```python
from build123d import *

# Parameters (mm, degrees)
BOSS_EXTRUDE1_DEPTH                       = 1.0668
CSK_FOR_6_FLAT_HEAD_MACHINE_SCREW_2_COUNT = 2
CSK_FOR_6_FLAT_HEAD_MACHINE_SCREW_2_PITCH = 75.64076181
CSK_FOR_6_FLAT_HEAD_MACHINE_SCREW_3_COUNT = 2
CSK_FOR_6_FLAT_HEAD_MACHINE_SCREW_3_PITCH = 28.085742046
CSK_FOR_6_FLAT_HEAD_MACHINE_SCREW_4_COUNT = 2
CSK_FOR_6_FLAT_HEAD_MACHINE_SCREW_4_PITCH = 31.783974209
CSK_FOR_6_FLAT_HEAD_MACHINE_SCREW_5_COUNT = 2
CSK_FOR_6_FLAT_HEAD_MACHINE_SCREW_5_PITCH = 85.183025791
CSK_FOR_6_FLAT_HEAD_MACHINE_SCREW_6_COUNT = 2
CSK_FOR_6_FLAT_HEAD_MACHINE_SCREW_6_PITCH = 53.560025791
CUT_EXTRUDE1_DEPTH                        = 78.375632316


with BuildPart() as part:
    # Sketch1 → Boss-Extrude1 (new body)
    with BuildSketch(Plane.XY):
        Polygon((-55.191374672, 13.731073684), (-72.605702167, -16.431426316), (75.603297833, -16.431426316), (58.188970339, 13.731073684), align=None)
    extrude(amount=BOSS_EXTRUDE1_DEPTH)

    # Sketch2 → CSK for #6 Flat Head Machine Screw (100)1 (revolve, cut)
    with BuildSketch(Plane(origin=(28.278810729, -11.668926316, 0), x_dir=(0, 1, 0), z_dir=(1, 0, 0))):
        Polygon((0, 0), (0, 1.0668), (1.89865, 1.0668), (1.89865, 1.380025208), (3.5433, 0), align=None)
    csk_for_6_flat_head_machine_screw_100 = revolve(axis=Axis((28.278810729, -11.668926316, -6.35), (0, 0, 1)), mode=Mode.SUBTRACT)

    # CSK for _6 Flat Head Machine Screw _ 2: CSK for #6 Flat Head Machine Screw (100)1 ×2
    with Locations(*[Vector(-0.9620606437367123, 0.27283569739479224, 0) * (i * CSK_FOR_6_FLAT_HEAD_MACHINE_SCREW_2_PITCH) for i in range(1, CSK_FOR_6_FLAT_HEAD_MACHINE_SCREW_2_COUNT)]):
        add(csk_for_6_flat_head_machine_screw_100, mode=Mode.SUBTRACT)

    # CSK for _6 Flat Head Machine Screw _ 3: CSK for #6 Flat Head Machine Screw (100)1 ×2
    with Locations(*[Vector(0.6782801027330659, 0.7348034446274878, 0) * (i * CSK_FOR_6_FLAT_HEAD_MACHINE_SCREW_3_PITCH) for i in range(1, CSK_FOR_6_FLAT_HEAD_MACHINE_SCREW_3_COUNT)]):
        add(csk_for_6_flat_head_machine_screw_100, mode=Mode.SUBTRACT)

    # CSK for _6 Flat Head Machine Screw _ 4: CSK for #6 Flat Head Machine Screw (100)1 ×2
    with Locations(*[(i * CSK_FOR_6_FLAT_HEAD_MACHINE_SCREW_4_PITCH, 0, 0) for i in range(1, CSK_FOR_6_FLAT_HEAD_MACHINE_SCREW_4_COUNT)]):
        add(csk_for_6_flat_head_machine_screw_100, mode=Mode.SUBTRACT)

    # CSK for _6 Flat Head Machine Screw _ 5: CSK for #6 Flat Head Machine Screw (100)1 ×2
    with Locations(*[(-i * CSK_FOR_6_FLAT_HEAD_MACHINE_SCREW_5_PITCH, 0, 0) for i in range(1, CSK_FOR_6_FLAT_HEAD_MACHINE_SCREW_5_COUNT)]):
        add(csk_for_6_flat_head_machine_screw_100, mode=Mode.SUBTRACT)

    # CSK for _6 Flat Head Machine Screw _ 6: CSK for #6 Flat Head Machine Screw (100)1 ×2
    with Locations(*[(-i * CSK_FOR_6_FLAT_HEAD_MACHINE_SCREW_6_PITCH, 0, 0) for i in range(1, CSK_FOR_6_FLAT_HEAD_MACHINE_SCREW_6_COUNT)]):
        add(csk_for_6_flat_head_machine_screw_100, mode=Mode.SUBTRACT)

    # Sketch4 → Cut-Extrude1 (cut, through all)
    with BuildSketch(Plane(origin=(0, 0, 0), x_dir=(-1, 0, 0), z_dir=(0, 0, -1))):
        Polygon((-65.308634086, 1.399454341), (-63.933818758, 0.605704341), (-56.355883234, 13.731073684), (-58.188970339, 13.731073684), align=None)
        Polygon((-68.483634086, -4.099806973), (-67.108818758, -4.893556973), (-73.770210729, -16.431426316), (-75.603297833, -16.431426316), align=None)
    cut_extrude1 = extrude(amount=-CUT_EXTRUDE1_DEPTH, mode=Mode.SUBTRACT)

    # Mirror1: Cut-Extrude1 across plane
    add(cut_extrude1.mirror(Plane.ZY.offset(-1.498797833)), mode=Mode.SUBTRACT)


solid = part.part
```
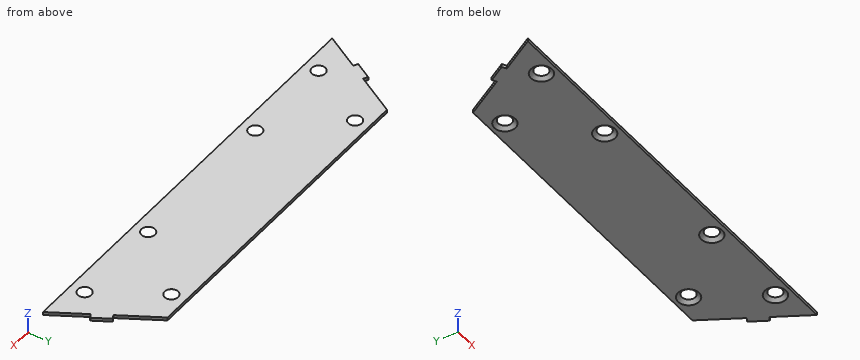
Model file for the job. Use its own axes, mm. Coordinates: 2 decimals unless noted, no trailing zeros. Loops run counter-clockwise (first coordinate to the right, second up) from the corner with the lowest first, then second, coordinate; pieces in that order, holes last. Notation, with made-up numbers: (82, -12.75) -> (100, -12.75) arc R20 ccw to (100, -6.75) -> close; hole circle Ø11 at (-5.75, 54). An arc over 180 degrees is marked (long way). Answer as a JSON object with one key per item and string values.
Q1. Flat gauge pin, fed straight in: P1, Ø1.5, axis at x = -28.5, y = 10, coming from the -Z side. Where does the tip first touch, or does it go through?
Report:
{"P1": "stops at z = 0"}
Q2. Cut at C-C (y = -1). List the corners of the cut face in (x, z), and give its area (3 significant figures).
Report:
{"outline": "(-63.7, 0) -> (66.69, 0) -> (66.69, 1.07) -> (-63.7, 1.07) -> close", "area": "139 mm2"}
Q3. Cut at B-B (y = 8.5). State how many separate pieces and enclosed holes the cut face has, and give its area (3 significant figures).
Report:
{"separate pieces": "3", "enclosed holes": "0", "area": "111 mm2"}
Q4. Cut at A-A (z = 0.6). List the corners of the cut face in (x, y).
Report:
{"outline": "(-70.77, -16.43) -> (73.77, -16.43) -> (67.11, -4.89) -> (68.48, -4.1) -> (65.31, 1.4) -> (63.93, 0.61) -> (56.36, 13.73) -> (-53.36, 13.73) -> (-60.94, 0.61) -> (-62.31, 1.4) -> (-65.49, -4.1) -> (-64.11, -4.89) -> close; hole circle Ø5.66 at (-56.9, -11.67); hole circle Ø5.66 at (-44.49, 8.97); hole circle Ø5.66 at (-25.28, -11.67); hole circle Ø5.66 at (28.28, -11.67); hole circle Ø5.66 at (47.33, 8.97); hole circle Ø5.66 at (60.06, -11.67)"}
Q5. Probe probe 1 along X at (y, z) = (9, 0.2); probe 2 along X at (y, z) = (-12, 0.85); probe 3 along X at (y, z) = (-13.5, 0.9). List the from-to ranges inside material, lowest first.
Report:
{"probe 1": "x = -56.09 to -47.8, -41.19 to 44.02, 50.63 to 59.09", "probe 2": "x = -68.21 to -59.41, -54.4 to -27.79, -22.77 to 25.77, 30.79 to 57.55, 62.57 to 71.21", "probe 3": "x = -69.08 to -58.56, -55.25 to -26.94, -23.62 to 26.62, 29.94 to 58.4, 61.72 to 72.08"}
